```python
from build123d import *

# Parameters (mm, degrees)
EXTRUDE1_DEPTH = 22


with BuildPart() as part:
    # Sketch1 → Revolve1 (revolve)
    with BuildSketch(Plane(origin=(0, 0, 0), x_dir=(1, 0, 0), z_dir=(0, 1, 0)), mode=Mode.PRIVATE) as revolve1_sk:
        Polygon((-72, 25), (72, 25), (152, 24.5), (153, 23.5), (153, 12.5), (157, 12.5), (158, 11.5), (158, 8.5), (180, 8.5), (180, 7), (209.5, 7), (210, 6.5), (210, 0), (-174, 0), (-174, 7.5), (-173, 8.5), (-158, 8.5), (-158, 11.5), (-157, 12.5), (-153, 12.5), (-153, 23.5), (-152, 24.5), align=None)
    revolve(revolve1_sk.sketch.rotate(Axis((-174, 0, 0), (1, 0, 0)), 180), axis=Axis((-174, 0, 0), (1, 0, 0)))  # turned: the seam where the file's is

    # Sketch2 → Extrude1 (cut, through all)
    with BuildSketch(Plane(origin=(0, 4, 0), x_dir=(-1, 0, 0), z_dir=(0, 1, 0))):
        with BuildLine():
            Line((-203.5, 2.5), (-192.5, 2.5))
            ThreePointArc((-192.5, 2.5), (-190, 0), (-192.5, -2.5))
            Line((-192.5, -2.5), (-203.5, -2.5))
            ThreePointArc((-203.5, -2.5), (-206, 0), (-203.5, 2.5))
        make_face()
    extrude(amount=EXTRUDE1_DEPTH, mode=Mode.SUBTRACT)


solid = part.part
```
Work out the finished part from the listing and answer in its coordinate system (mm). A direction names the side the tool comes from. Give positions to 0.01 mm unless a question says otherwise; leave off trailing zeros. Order: outer loops, then holes, each group sorted by start corner. A loop starts at its lowest first (then second) coordinate and runs counter-clockwise, first axis right, second up. Notation, with made-up numbers: M -36.75,40.25 L -12.75,40.25 A23 cw -12.75,60.25 Z; hole C 60,89 d8. An arc over 180 degrees is marked long. Return JSON: item names as keys, results as strings.
1) A tool of negligible diameter and unlimited length cuts with its end or side. For faces 1 (the cylindrical face through (-165.395, -8.428, -1.107)), 2 (the flat face through (180, -7, 2)), 3 (the flat face through (210, 0, 0)), from which of +Z, -Z, +X, -X, +Y, -Y can it reach the whole face along a straight path? Write none if from no direction.
Resolved:
{"face 1": "-X", "face 2": "+X", "face 3": "+Z, -Z, +X, +Y, -Y"}
2) Section B-B, the plane x = 16 is taken. Write down the section's boundary in (y, z), plus the area to 3 significant figures.
Resolved:
{"outline": "C 0,0 d50", "area": "1,960 mm^2"}
3) Straight lines are drawn through the part: line 1 along X through (y, z) = (14, 9); line 2 along Z through (x, y) = (27, 1); line 3 along Z through (x, y) = (128, 4). For each, find the intervals that lie inside material, in ascending order. Write a range as [from, to].
Resolved:
{"line 1": "[-153, 153]", "line 2": "[-24.98, 24.98]", "line 3": "[-24.32, 24.32]"}
4) Section A-A, the plane x = 80 is taken. Write down the section's boundary in (y, z).
Resolved:
{"outline": "C 0,0 d49.9"}
5) Each of these flat-tipped pins is pushed along its axis until it touches: pin 1 (1.3 mm diameter, centred on x = 197, y = 5, fed in from +Z); pin 2 (8 mm diameter, centred on y = 14, z = 11.5, fed in from +X); pin 3 (12 mm diameter, centred on x = 88, z = -4, fed in from +Y). Where does it stop, or does it pass through?
Resolved:
{"pin 1": "z = 5.48", "pin 2": "x = 153", "pin 3": "y = 24.93"}
